Verification items for the finished model (mm, model axes). Coordinates: 2 decimals unless noted, no trailing zeros. Order: outer loops, then holes, each group sorted by start corner. A loop starts at its lowest first (then second) coordinate and runs counter-clockwise, first axis right, second up. Notation, with made-up numbers: (60.5, -17) -> (102.5, -17) arc R20 ccw to (102.5, 21) -> close; hole circle Ø1 at (38, 28). An arc over 180 degrees is marked (long way). Use CSV: the item, a comma, the result in double quotes. Start each with the question number.
1) Scan lines: line 1 along X through (y, z) = (-8.5, 19); line 2 along X through (y, z) = (8.75, -53.5); line 3 along Z through (x, y) = (-30.75, 10.25). Record each from-to range of solid material in increasing order.
2) Release check for a two-part mould opening along Z. For faces 1 (the flat face through (-31, 8, -110)), 2 (the cylindrical face through (-30.092, 9.601, -108.028)), 3 (the conical face through (-32.15, 10.15, -104.32)) record: released by +Z, released by -Z, zero draft, split by the parting line, or undercut.
3) Sectioned sample at A-A on z = -78.5. Record the boundary of the cut face in (x, y), then the cut area to 3 significant figures.
4) Go/stop test with flat-tipped pins: pin 1 (12 mm diameter, centred on y = -5, z = 53.5, fed in from +X); pin 2 (5 mm diameter, centred on x = -33.5, z = 28, fed in from +Y). Record where each tip stops, or that it passes through.
from build123d import *

# Parameters (mm, degrees)
CYLINDER068_R               = 1
CYLINDER068_DEPTH           = 68
CYLINDER068_ROLL_ANGLE      = 13.101784
CYLINDER068_PITCH_ANGLE     = -8.567577
CYLINDER068_PLACEMENT_ANGLE = 13.101784
CYLINDER054_R               = 1
CYLINDER054_DEPTH           = 50
CYLINDER065_R               = 1
CYLINDER065_DEPTH           = 87
CYLINDER052_R               = 2
CYLINDER052_DEPTH           = 4
CYLINDER053_R               = 1
CYLINDER053_DEPTH           = 8


with BuildPart() as cylindre064:
    # Cylinder068 → Cylinder068 (new body)
    with BuildSketch(Plane.XY):
        Circle(CYLINDER068_R)
    extrude(amount=CYLINDER068_DEPTH)


with BuildPart() as cylindre064_1:
    # Cylinder068 roll: moved
    add(cylindre064.part.rotate(Axis((0, 0, 0), (1, 0, 0)), CYLINDER068_ROLL_ANGLE))


with BuildPart() as cylindre064_2:
    # Cylinder068 pitch: moved
    add(cylindre064_1.part.rotate(Axis((0, 0, 0), (0, 1, 0)), CYLINDER068_PITCH_ANGLE))


with BuildPart() as cylindre064_3:
    # Cylinder068 placement: moved
    add(cylindre064_2.part.moved(Location((-32, 9, -55))).rotate(Axis((-32, 9, -55), (0, 0, 1)), CYLINDER068_PLACEMENT_ANGLE))


with BuildPart() as fusion031:
    # Cylinder054 → Cylinder054 (new body)
    with BuildSketch(Plane(origin=(-32, 9, -104), x_dir=(1, 0, 0), z_dir=(0, 0, 1))):
        Circle(CYLINDER054_R)
    extrude(amount=CYLINDER054_DEPTH)

    # Fusion031: union Cylindre064
    add(cylindre064_3.part)


with BuildPart() as fusion032:
    # Cylinder065 → Cylinder065 (new body)
    with BuildSketch(Plane(origin=(-38, -8.4, 10), x_dir=(1, 0, 0), z_dir=(0, 0, 1))):
        Circle(CYLINDER065_R)
    extrude(amount=CYLINDER065_DEPTH)

    # Fusion032: union Fusion031
    add(fusion031.part)


with BuildPart() as obj1:
    # Cone001 → Cone001 (revolve)
    with BuildSketch(Plane(origin=(-32, 9, -106), x_dir=(1, 0, 0), z_dir=(0, -1, 0))):
        Polygon((0, 0), (2, 0), (1, 2), (0, 2), align=None)
    revolve(axis=Axis((-32, 9, -106), (0, 0, 1)))


with BuildPart() as fusion033:
    # Cylinder052 → Cylinder052 (new body)
    with BuildSketch(Plane(origin=(-32, 9, -110), x_dir=(1, 0, 0), z_dir=(0, 0, 1))):
        Circle(CYLINDER052_R)
    extrude(amount=CYLINDER052_DEPTH)

    # Fusion026: union obj1
    add(obj1.part)

    # Fusion033: union Fusion032
    add(fusion032.part)


with BuildPart() as fusion034:
    # Cylinder053 → Cylinder053 (new body)
    with BuildSketch(Plane(origin=(-32, 9, -116), x_dir=(1, 0, 0), z_dir=(0, 0, 1))):
        Circle(CYLINDER053_R)
    extrude(amount=CYLINDER053_DEPTH)

    # Fusion034: union Fusion033
    add(fusion033.part)


solid = fusion034.part
Answers follow:
1,line 1,"x = -38.99 to -37.01"
1,line 2,"x = -33.13 to -31.14"
1,line 3,"z = -110 to -105.54"
2,face 1,"released by -Z"
2,face 2,"zero draft"
2,face 3,"undercut"
3,outline,"circle Ø2 at (-32, 9)"
3,area,"3.14 mm²"
4,pin 1,"stops at x = -37"
4,pin 2,"passes through"
